```python
from build123d import *

# Parameters (mm, degrees)
F0_R     = 27
F1_DEPTH = 1.5
F2_R     = 1.49999


# Not quite as in the source:
# - a fillet or chamfer is up to 0.001 mm smaller than in the source, because OpenCascade refuses the exact size


with BuildPart() as f1:
    # F0 (on Front) → F1 (new body, symmetric)
    with BuildSketch(Plane.XZ):
        with BuildLine():
            Line((150, 0), (-150, 0))
            Line((-150, 0), (-150, -3))
            Line((-150, -3), (-13.0766968306, -3))
            ThreePointArc((-13.0766968306, -3), (0, -60), (13.0766968306, -3))
            Line((13.0766968306, -3), (150, -3))
            Line((150, -3), (150, 0))
        make_face()
        with Locations((0, -30)):
            Circle(F0_R, mode=Mode.SUBTRACT)
    extrude(amount=F1_DEPTH, both=True)

    # F2 (radius 1.5 in the source; OpenCascade refuses exactly that, so slightly less here)
    f2_edges = [f1.edges().sort_by_distance(p)[0] for p in [
        (-81.538348, -1.5, -3),
        (0, -1.5, 0),
        (0, 1.5, 0),
        (-81.538348, 1.5, -3),
        (81.538348, -1.5, -3),
        (81.538348, 1.5, -3),
    ]]
    fillet(f2_edges, radius=F2_R)


solid = f1.part
```
Could you check a few things on this model? Use its own coordinates, in mm. Give positions to 0.01 mm unless a question says otherwise; leave off trailing zeros. Write each loop counter-clockwise with the first axis right and the second up, starting at its lowest first coordinate (ties: lowest second). Pieces come first, ordered by that corner, then holes. Notation, with made-up numbers: (74, 58) - (111, 58) arc R28 cw to (111, 88) - close; hole circle Ø1 at (-24, -15.5). An arc over 180 degrees is marked (long way). One line per item, written item: value. Start each with the question number.
Item 1: Imagine slicing it at D-D, the plane z = -13.5. List the corners of the cut face in (x, y) for me, and give its area (3 significant figures).
Item 2: If we mould it in two halves opening along X, with no side actions, what happens to faces 1 (the face through (-3.51, 0.02, -3.23)), 2 (the face through (-23, -1.5, -15))? For each: +X half, -X half, draft (parallel to the pull), parting line (faces both ways), or undercut.
Item 3: Please list where these lines run through material, in increasing order: line 1 (X direction, y = -0.8, z = -28.5); line 2 (Z direction, x = 0, y = -0.25); line 3 (Z direction, x = -23, y = 0.65). Write a range as from..to.
Item 4: Imagine slicing it at A-A, the plane z = -30. List the corners of the cut face in (x, y) for me.
Item 5: I'm going to push a flat-ended pin straight in: pin 1 (1 mm diameter, centred on y = 0.5, z = -39.5, fed in from -X). Where does the tip first touch, or does it pass through?
Geometry says:
1. outline: (-25.05, -1.5) - (-21.37, -1.5) - (-21.37, 1.5) - (-25.05, 1.5) - close; (21.37, -1.5) - (25.05, -1.5) - (25.05, 1.5) - (21.37, 1.5) - close
1. area: 22.1 mm^2
2. face 1: undercut
2. face 2: draft
3. line 1: -29.96..-26.96, 26.96..29.96
3. line 2: -60..-57, -3..-0.02
3. line 3: -49.26..-44.14, -15.86..-10.74, -2.85..-0.15
4. outline: (-30, -1.5) - (-27, -1.5) - (-27, 1.5) - (-30, 1.5) - close; (27, -1.5) - (30, -1.5) - (30, 1.5) - (27, 1.5) - close
5. pin 1: x = -28.62
